Check sheet for the modelled part. Datum: model origin and axes. Units: mm. A direction names the side the tool comes from. Round coordinates to 2 decimals unless told otherwise and drop trailing zeros. Order: outer loops, then holes, each group sorted by start corner. A loop starts at its lowest first (then second) coordinate and runs counter-clockwise, first axis right, second up. Notation, with made-up numbers: (-7.75, -17.5) -> (0.25, -17.5) arc R20 cw to (0.25, -5.5) -> close; hole circle Ø5 at (74, -21.5). An arc over 180 degrees is marked (long way). Answer in a Markdown table with one row per item.
from build123d import *

# Parameters (mm, degrees)
BOSS_EXTRUDE1_DEPTH = 5.08
SKETCH3_W           = 11.43
SKETCH3_H           = 11.43
BOSS_EXTRUDE2_DEPTH = 1.27
SKETCH5_R           = 4.961688794
SKETCH5_R_2         = 0.865135847
BOSS_EXTRUDE3_DEPTH = 1.27


with BuildPart() as part:
    # Sketch1 → Boss-Extrude1 (new body)
    with BuildSketch(Plane(origin=(0, 0, 0), x_dir=(1, 0, 0), z_dir=(0, 1, 0))):
        Polygon((-19.516726296, 9.048937426), (5.883273704, 9.048937426), (5.883273704, 5.480342385), (9.058273704, 5.480342385), (9.058273704, -14.839657615), (-22.691726296, -14.839657615), (-22.691726296, 5.480342385), (-19.516726296, 5.480342385), align=None)
    extrude(amount=BOSS_EXTRUDE1_DEPTH)

    # Sketch3 → Boss-Extrude2 (add)
    with BuildSketch(Plane(origin=(0, 5.08, 0), x_dir=(1, 0, 0), z_dir=(0, 1, 0))):
        with Locations((-6.816726296, -4.154305268)):
            Rectangle(SKETCH3_W, SKETCH3_H)
    extrude(amount=BOSS_EXTRUDE2_DEPTH)

    # Sketch5 → Boss-Extrude3 (add)
    with BuildSketch(Plane(origin=(0, 6.35, 0), x_dir=(1, 0, 0), z_dir=(0, 1, 0))):
        with Locations(Location((-7.009181054, -4.258692446, 0), (0, 0, 270))):
            Circle(SKETCH5_R)
        with Locations(Location((-7.009181054, -4.258692446, 0), (0, 0, 270))):
            Circle(SKETCH5_R_2, mode=Mode.SUBTRACT)
    extrude(amount=BOSS_EXTRUDE3_DEPTH)


solid = part.part
Item 1: Cross-section at A-A (y = 2). Record the boundary of the cut face in (x, z).
Result sheet:
| item | result |
|---|---|
| outline | (-22.69, -5.48) -> (-19.52, -5.48) -> (-19.52, -9.05) -> (5.88, -9.05) -> (5.88, -5.48) -> (9.06, -5.48) -> (9.06, 14.84) -> (-22.69, 14.84) -> close |
Item 2: Scan lines: line 1 (Y direction, x = -19.5, z = -4); line 2 (Z direction, x = -5.5, y = 6); line 3 (Z direction, x = 8.5, y = 4.25). Record each from-to range of solid material in increasing order. Write a range as [from, to].
Result sheet:
| item | result |
|---|---|
| line 1 | y = [0, 5.08] |
| line 2 | z = [-1.56, 9.87] |
| line 3 | z = [-5.48, 14.84] |
Item 3: Cross-section at D-D (x = -11). Record the boundary of the cut face in (y, z).
Result sheet:
| item | result |
|---|---|
| outline | (0, -9.05) -> (5.08, -9.05) -> (5.08, -1.56) -> (6.35, -1.56) -> (6.35, 1.31) -> (7.62, 1.31) -> (7.62, 7.21) -> (6.35, 7.21) -> (6.35, 9.87) -> (5.08, 9.87) -> (5.08, 14.84) -> (0, 14.84) -> close |
Item 4: Set-up check for faces 5 (the flat face through (7, 3, -5.48)), 6 (the flat face through (-12.532, 6, 4)), 7 (the flat face through (-1.102, 6, 4)), 8 (the flat face through (-21, 3, -5.48)), 9 (the flat face through (-7, 6.35, -1)): record each of +Z, -Z, +X, -X, +Y, -Y from which the full face is reachable in a straight line by a thin tool's end or side.
Result sheet:
| item | result |
|---|---|
| face 5 | -Z, +X, +Y, -Y |
| face 6 | +Z, -Z, -X, +Y |
| face 7 | +Z, -Z, +X, +Y |
| face 8 | -Z, -X, +Y, -Y |
| face 9 | +Y |
Item 5: Cross-section at B-B (x = -4). Record the boundary of the cut face in (y, z), and give its area (3 significant figures).
Result sheet:
| item | result |
|---|---|
| outline | (0, -9.05) -> (5.08, -9.05) -> (5.08, -1.56) -> (6.35, -1.56) -> (6.35, 0.31) -> (7.62, 0.31) -> (7.62, 8.2) -> (6.35, 8.2) -> (6.35, 9.87) -> (5.08, 9.87) -> (5.08, 14.84) -> (0, 14.84) -> close |
| area | 146 mm^2 |
Item 6: Depth check by flat-ended pin: P1, Ø1, axis at x = 6.5, y = 3.5, coming from the -Z side; P2, Ø1.8, axis at y = 2.5, z = -7, coming from the +X side; P3, Ø0.9, axis at x = -7, z = 4, coming from the +Y side. Enter the tip coordinate at first touch or a pass-through.
Result sheet:
| item | result |
|---|---|
| P1 | stops at z = -5.48 |
| P2 | stops at x = 5.88 |
| P3 | stops at y = 6.35 |
Item 7: Cross-section at C-C (z = 11.25). Record the boundary of the cut face in (x, y), and give its area (3 significant figures).
Result sheet:
| item | result |
|---|---|
| outline | (-22.69, 0) -> (9.06, 0) -> (9.06, 5.08) -> (-22.69, 5.08) -> close |
| area | 161 mm^2 |
Item 8: Mould release check, pull along Z, two halves, no side actions. Record for faces 1 (the cylindrical face through (-3.66, 6.98, 0.6)), 2 (the flat face through (5.883, 3, -7)), 3 (the flat face through (-7, 6.35, 4)), 4 (the flat face through (-7, 6, 9.869)): pulls with the +Z half, pulls with the -Z half, needs draft (parallel to the pull), parting line crosses it, or undercut.
Result sheet:
| item | result |
|---|---|
| face 1 | parting line crosses it |
| face 2 | needs draft |
| face 3 | undercut |
| face 4 | pulls with the +Z half |
